from build123d import *

# Parameters (mm, degrees)
F1_DEPTH = 10
F0_W     = 10
F0_H     = 80
F2_DEPTH = 25


with BuildPart() as f1:
    # F0 (on Top) → F1 (new body)
    with BuildSketch(Plane.XY):
        Polygon((-4.978042, 40), (-40, 40), (-40, 5), (-50, 5), (-50, 15), (-60, 15), (-60, -15), (-50, -15), (-50, -5), (-40, -5), (-40, -40), (-5, -40), (-5, -50), (-15, -50), (-15, -60), (15, -60), (15, -50), (5, -50), (5, -40), (40, -40), (40, 40), (6.021958, 40), (6.021958, 30.516871), (16.021958, 30.516871), (16.021958, 19.516871), (-14.978042, 19.516871), (-14.978042, 30.516871), (-4.978042, 30.516871), align=None)
    extrude(amount=F1_DEPTH)

    # F0 (on Top) → F2 (join)
    with BuildSketch(Plane.XY):
        with Locations((45, 0)):
            Rectangle(F0_W, F0_H)
    extrude(amount=F2_DEPTH)


solid = f1.part
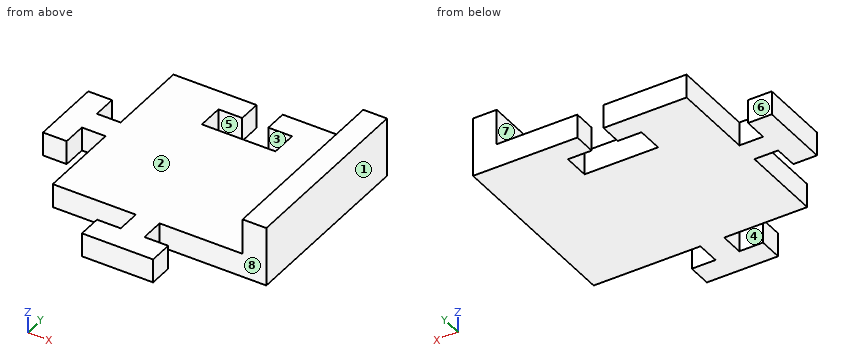
Design review of the part built by this model. Coordinates are the model's own, in mm. Face numbers are marked on the shaded views. A direction names the side the tool comes from. Round coordinates to 2 decimals unless told otherwise and drop trailing zeros. Write each loop counter-clockwise with the first axis right and the second up, starting at its lowest first coordinate (ties: lowest second). Pieces come first, ordered by that corner, then holes. Notation, with made-up numbers: (-3, 71.5) - (37, 71.5) arc R23 ccw to (37, 104.5) - close; hole circle Ø8 at (-22.75, 15.5). An arc over 180 degrees is marked (long way). Use a Markdown table: item, result. Add a question column.
1. We need section C-C (z = 7.25). State the section outline as (x, y) points.
2. We need section D-D (y = -7). State the section outline as (x, z) points.
3. We need section A-A (y = 27.5). State the section outline as (x, z) points.
4. For the marked faces 4, 5, 6, 7 and 8, list the 3-axis set-ups (+Z, -Z, +X, -X, +Y, -Y) from which the entire face can be reached by the end or side of a thin tool; tool diameter is ignored.
5. Clearance check with flat-ended pins moving along their axes: pin 1 (8 mm diameter, centred on x = -21, z = 4, fed in from -Y); pin 2 (5 mm diameter, centred on y = -56.5, z = 3.5, fed in from +X); pin 3 (6 mm diameter, centred on x = -13, y = 21.5, fed in from +Z). State where each tip first meets the part, or that it passes through.
6. We need section B-B (x = 9.5). State the section outline as (y, z) points.
7. Wall thickness on probe 1 along Y at (x, z) = (-9, 4.5); probe 2 along X at (y, z) = (19, 14.75); probe 3 along Z at (x, y) = (-4, 14): over which ranges is each line inside the solid? List them lowest first.
8. Mouldability with a two-part tool opening along X and no side actions: class the marked faces 1, 2 and 3 as +X half, -X half, draft (parallel to the pull), parting line (faces both ways), or undercut.
Output:
| question | item | result |
|---|---|---|
| 1 | outline | (-60, -15) - (-50, -15) - (-50, -5) - (-40, -5) - (-40, -40) - (-5, -40) - (-5, -50) - (-15, -50) - (-15, -60) - (15, -60) - (15, -50) - (5, -50) - (5, -40) - (50, -40) - (50, 40) - (6.02, 40) - (6.02, 30.52) - (16.02, 30.52) - (16.02, 19.52) - (-14.98, 19.52) - (-14.98, 30.52) - (-4.98, 30.52) - (-4.98, 40) - (-40, 40) - (-40, 5) - (-50, 5) - (-50, 15) - (-60, 15) - close |
| 2 | outline | (-60, 0) - (-50, 0) - (-50, 10) - (-60, 10) - close; (-40, 0) - (50, 0) - (50, 25) - (40, 25) - (40, 10) - (-40, 10) - close |
| 3 | outline | (-40, 0) - (-14.98, 0) - (-14.98, 10) - (-40, 10) - close; (16.02, 0) - (50, 0) - (50, 25) - (40, 25) - (40, 10) - (16.02, 10) - close |
| 4 | face 4 | +Z, -Z, -X |
| 4 | face 5 | +Z, -Z |
| 4 | face 6 | +Z, -Z, -X, +Y |
| 4 | face 7 | +Z, -X, +Y, -Y |
| 4 | face 8 | +Z, -Z, +X |
| 5 | pin 1 | stops at y = -40 |
| 5 | pin 2 | stops at x = 15 |
| 5 | pin 3 | stops at z = 10 |
| 6 | outline | (-60, 0) - (-50, 0) - (-50, 10) - (-60, 10) - close; (-40, 0) - (19.52, 0) - (19.52, 10) - (-40, 10) - close; (30.52, 0) - (40, 0) - (40, 10) - (30.52, 10) - close |
| 7 | probe 1 | y = -60 to -50, -40 to 19.52, 30.52 to 40 |
| 7 | probe 2 | x = 40 to 50 |
| 7 | probe 3 | z = 0 to 10 |
| 8 | face 1 | +X half |
| 8 | face 2 | draft |
| 8 | face 3 | undercut |
